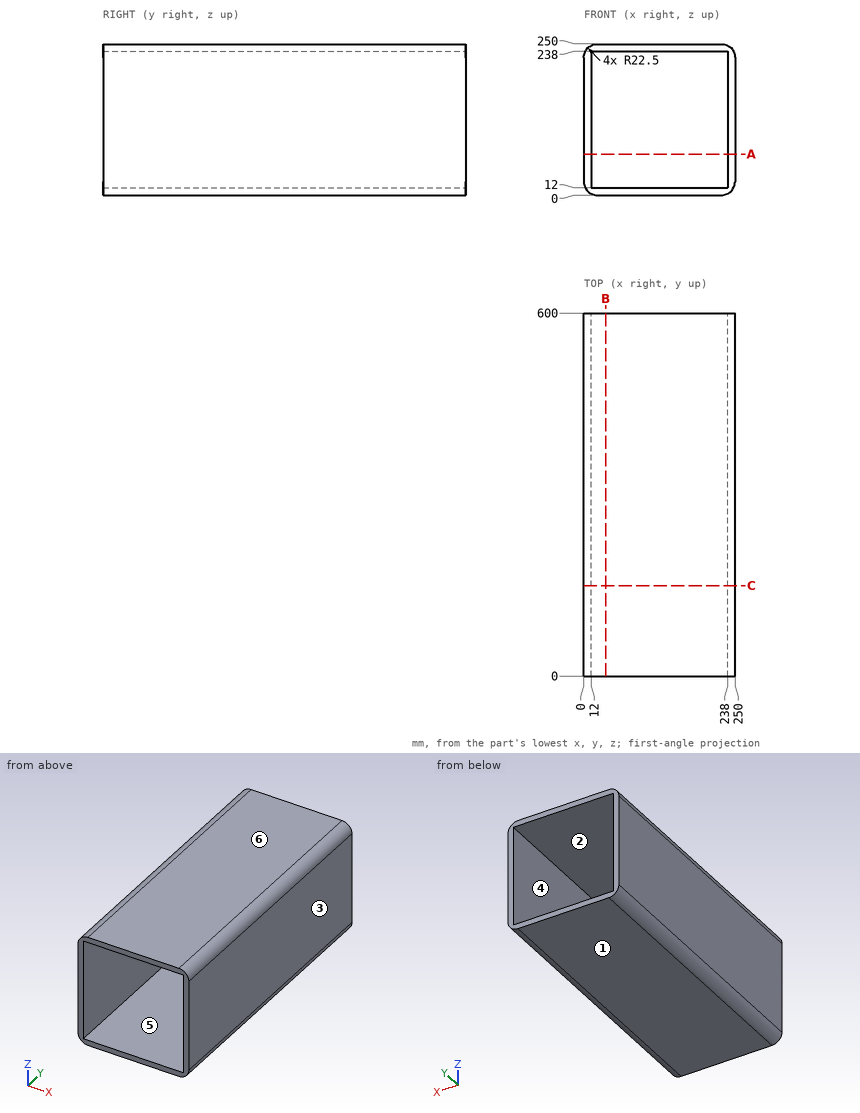
Source: three-view drawing plus pictorial views. Frame: mm from the lowest corner of the part. A direction names the side the tool comes from. Give positions to 0.01 mm unless a question says otherwise; leave off trailing zeros. Write each loop counter-clockwise with the first axis right and the second up, starting at its lowest first coordinate (ties: lowest second). Pieces come first, ordered by that corner, then holes. Notation, with made-up numbers: (-30, 25) - (-14, 25) arc R26 cw to (-14, 50) - close; hole circle Ø7 at (46.5, 6). An arc over 180 degrees is marked (long way). Write item = value, one per line. Start each with the question number.
1. Section query A-A, the plane z = 68. Output: boundary loops of the cut face in (x, y), then the cut area to 3 significant figures.
2. Section query B-B, the plane x = 36. Output: boundary loops of the cut face in (y, z).
3. Access query for the marked faces 5 and 6. Directions: +Z, -Z, +X, -X, +Y, -Y. A direction counts if a zero-diameter tool reaches every point of the face in a straight line with its end or side. Return the directions, or none.
4. Mould query, pull axis X, two halves, no side actions, for the marked faces 1, 2, 3 and 4. Classes: released by +X, released by -X, zero draft, split by the parting line, or undercut.
5. Ray query, L1, parallel to X at y = 332.5, z = 30.5; L2, parallel to X at y = 565, z = 229. Return the intervals inside material, ascending.
6. Section query C-C, the plane y = 149.5. Output: boundary loops of the cut face in (x, z).
Check sheet entries:
q1.outline = (0, 0) - (12, 0) - (12, 600) - (0, 600) - close; (238, 0) - (250, 0) - (250, 600) - (238, 600) - close
q1.area = 14,400 mm2
q2.outline = (0, 0) - (600, 0) - (600, 12) - (0, 12) - close; (0, 238) - (600, 238) - (600, 250) - (0, 250) - close
q3.face_5 = +Y, -Y
q3.face_6 = +Z, +X, -X, +Y, -Y
q4.face_1 = zero draft
q4.face_2 = undercut
q4.face_3 = released by +X
q4.face_4 = undercut
q5.L1 = 0 to 12, 238 to 250
q5.L2 = 0.05 to 12, 238 to 249.95
q6.outline = (0, 22.5) arc R22.5 ccw to (22.5, 0) - (227.5, 0) arc R22.5 ccw to (250, 22.5) - (250, 227.5) arc R22.5 ccw to (227.5, 250) - (22.5, 250) arc R22.5 ccw to (0, 227.5) - close; hole (12, 12) - (238, 12) - (238, 238) - (12, 238) - close
